For this review, take the finished solid that the model builds, in its own axes (mm). A direction names the side the tool comes from. Give positions to 0.01 mm unless a question says otherwise; leave off trailing zeros. Loops run counter-clockwise (first coordinate to the right, second up) from the corner with the lowest first, then second, coordinate; pieces in that order, holes last. Notation, with made-up numbers: (40.25, 5.5) -> (63.25, 5.5) arc R32 ccw to (63.25, 31.5) -> close; hole circle Ø2 at (81, 4). An arc over 180 degrees is marked (long way). Answer as CSV lines item,"result". Start each with the question number.
Item 1: Add section C-C on y = 9.25. State the section outline as (x, z) points, plus the area to 3 significant figures.
Item 2: Machinability: for faces 1 (the face through (113, 13, -23.812)), 2 (the face through (230, 1, -13)), which of the approach directions +Z, -Z, +X, -X, +Y, -Y give a long, thin tool a straight path to every point of the face, cutting with its end or side? Answer none if there is none.
Item 3: The part is to be moulded in two halves that separate along Z. For faces 3 (the face through (0, 1, -13)), 4 (the face through (113, 1.588, -13)), 5 (the face through (113, 13, 0)), say which applies: +Z half, -Z half, draft (parallel to the pull), parting line (faces both ways), or undercut.
Item 4: For L1, parallel to Z at x = 122, y = 2.25; L2, parallel to Y at x = 83, z = -4.5, list the stretches that pass through material, from the lowest coordinate up. Write a range as from..to.
Item 5: Add section B-B on x = 134. State the section outline as (y, z) points, plus the area to 3 significant figures.
Item 6: Add section A-A on z = -15.75. State the section outline as (x, y) points, plus the area to 3 significant figures.
Autodesk Inventor part; units mm, degrees
ref_plane "YZ Plane" through (0, 0, 0) normal (1, 0, 0) x (0, 1, 0)
ref_plane "XZ Plane" through (0, 0, 0) normal (0, 1, 0) x (-1, 0, 0)
ref_plane "XY Plane" through (0, 0, 0) normal (0, 0, 1) x (1, 0, 0)
sketch "Sketch1" plane through (0, 0, 0) normal (1, 0, 0) x (0, 1, 0)
  line L0 (0, 0) -> (25.4, 0)
  line L1 (25.4, 0) -> (25.4, -25.4)
  line L2 (25.4, -25.4) -> (0, -25.4)
  line L3 (0, -25.4) -> (0, 0)
  line L4 (23.8125, -23.8125) -> (23.8125, -1.5875)
  line L5 (23.8125, -1.5875) -> (1.5875, -1.5875)
  line L6 (1.5875, -1.5875) -> (1.5875, -23.8125)
  line L7 (1.5875, -23.8125) -> (23.8125, -23.8125)
  dimension "d0" = 25.4
  dimension "d1" = 25.4
  dimension "d2" = 1.5875
extrude "Extrusion1" add sketch "Sketch1" along normal blind 230
sketch "Sketch2" plane through (0, 25.4, 0) normal (0, 1, 0) x (1, 0, 0)
  point P0 (0, 0)
properties part number "HOrizontal_Beam_Short"
Computed values:
1,outline,"(0, -25.4) -> (230, -25.4) -> (230, -23.81) -> (0, -23.81) -> close; (0, -1.59) -> (230, -1.59) -> (230, 0) -> (0, 0) -> close"
1,area,"730 mm²"
2,face 1,"+X, -X"
2,face 2,"+Z, -Z, +X, +Y, -Y"
3,face 3,"draft"
3,face 4,"undercut"
3,face 5,"+Z half"
4,L1,"-25.4..-23.81, -1.59..0"
4,L2,"0..1.59, 23.81..25.4"
5,outline,"(0, -25.4) -> (25.4, -25.4) -> (25.4, 0) -> (0, 0) -> close; hole (1.59, -23.81) -> (23.81, -23.81) -> (23.81, -1.59) -> (1.59, -1.59) -> close"
5,area,"151 mm²"
6,outline,"(0, 0) -> (230, 0) -> (230, 1.59) -> (0, 1.59) -> close; (0, 23.81) -> (230, 23.81) -> (230, 25.4) -> (0, 25.4) -> close"
6,area,"730 mm²"
